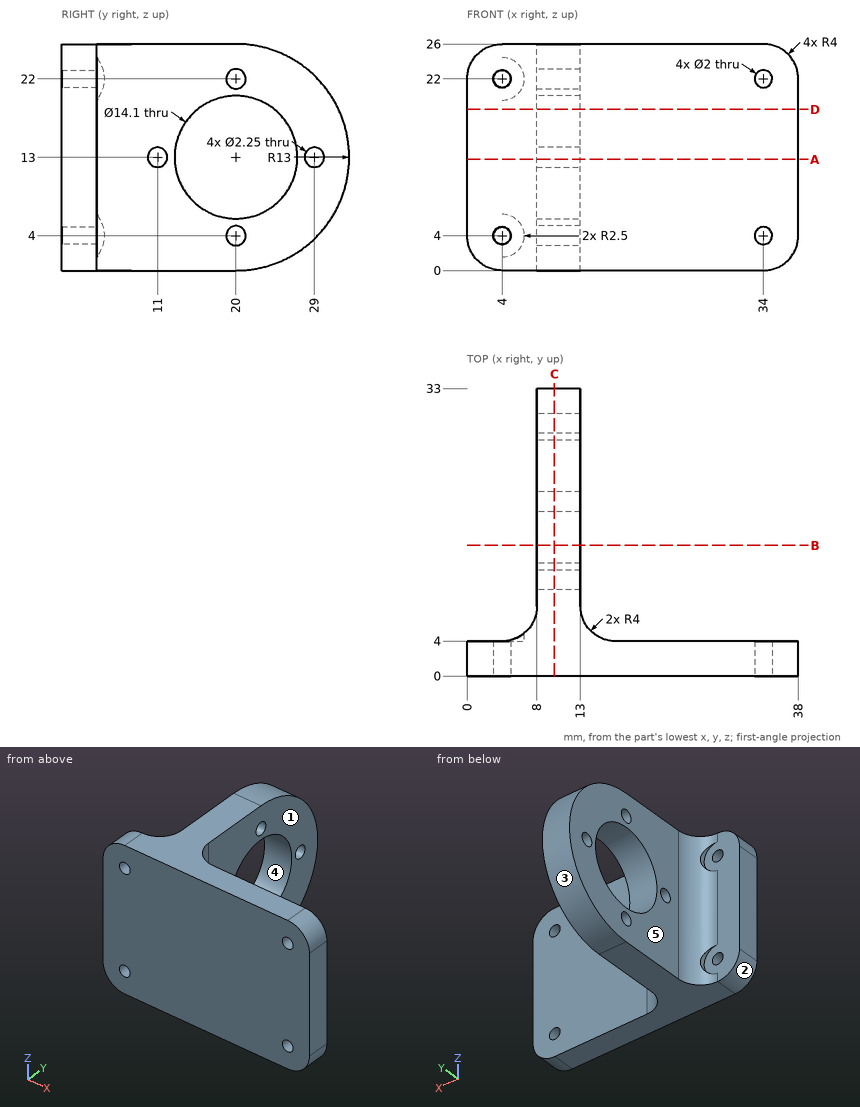
Here's the drawing with two shaded views (mm, measured from the low corner). I have some questions. A direction names the side the tool comes from. Round coordinates to 2 decimals unless told otherwise and drop trailing zeros. Order: outer loops, then holes, each group sorted by start corner. A loop starts at its lowest first (then second) coordinate and runs counter-clockwise, first axis right, second up. Notation, with made-up numbers: (85.5, 57) -> (98.5, 57) arc R17 cw to (98.5, 88) -> close; hole circle Ø1 at (16.25, 41.5). An arc over 180 degrees is marked (long way). Write each question's results on one line, items separated by ' | '. Start each with the question number.
Item 1: If we section it at C-C, the plane x = 10: Write out the boundary of the cut face in (y, z) (3 decimals), then the cut area to 3 significant figures.
Item 2: Thinking about a two-plate mould opening in Z: for the marked faces 3, 4 and 5, which applies, +Z half, -Z half, draft (parallel to the pull), parting line (faces both ways), or undercut?
Item 3: Which directions (+Z, -Z, +X, -X, +Y, -Y) give clear straight access to the entire face, cutting with the end or side of a thin tool? Please do the marked faces 1 and 2.
Item 4: Will these pins go through, and if not, where does the flat tip stop? pin 1 (10.5 mm diameter, centred on x = 23.5, z = 8.5, fed in from +Y); pin 2 (1.8 mm diameter, centred on x = 34, z = 4, fed in from -Y); pin 3 (3 mm diameter, centred on x = 10.5, z = 7.5, fed in from +Y); pin 4 (3 mm diameter, centred on y = 29.5, z = 17, fed in from -X).
Item 5: If we section it at D-D, the plane z = 18.5: Write out the boundary of the cut face in (x, y), then the cut area to 3 significant figures.
Item 6: If we section it at B-B, the plane y = 15: Write out the boundary of the cut face in (x, z), then the cut area to 3 significant figures.
Item 7: If we section it at A-A, the plane z = 12.75: Write out the boundary of the cut face in (x, y), then the cut area to 3 significant figures.
Item 8: Please list where these lines run through material, in increasing order: L1, parallel to Y at x = 10.5, z = 13 (3 decimals); L2, parallel to Y at x = 10, z = 12.5; L3, parallel to X at y = 26, z = 18.5.
Results:
1) outline: (0, 0) -> (20, 0) arc R13 ccw to (20, 26) -> (0, 26) -> close; hole circle Ø2.25 at (11, 13); hole circle Ø14.1 at (20, 13); hole circle Ø2.25 at (20, 4); hole circle Ø2.25 at (20, 22); hole circle Ø2.25 at (29, 13) | area: 613 mm2
2) face 3: parting line | face 4: undercut | face 5: draft
3) face 1: +Z, -Z, +X, +Y | face 2: -Z, -X, +Y, -Y
4) pin 1: stops at y = 4 | pin 2: passes through | pin 3: stops at y = 32.37 | pin 4: stops at x = 8
5) outline: (0, 0) -> (38, 0) -> (38, 4) -> (17, 4) arc R4 cw to (13, 8) -> (13, 15.59) -> (8, 15.59) -> (8, 8) arc R4 cw to (4, 4) -> (0, 4) -> close; (8, 24.41) -> (13, 24.41) -> (13, 31.78) -> (8, 31.78) -> close | area: 254 mm2
6) outline: (8, 0) -> (13, 0) -> (13, 8.03) -> (8, 8.03) -> close; (8, 17.97) -> (13, 17.97) -> (13, 26) -> (8, 26) -> close | area: 80.3 mm2
7) outline: (0, 0) -> (38, 0) -> (38, 4) -> (17, 4) arc R4 cw to (13, 8) -> (13, 9.9) -> (8, 9.9) -> (8, 8) arc R4 cw to (4, 4) -> (0, 4) -> close; (8, 12.1) -> (13, 12.1) -> (13, 12.95) -> (8, 12.95) -> close; (8, 27.05) -> (13, 27.05) -> (13, 27.9) -> (8, 27.9) -> close; (8, 30.1) -> (13, 30.1) -> (13, 33) -> (8, 33) -> close | area: 211 mm2
8) L1: y = 0 to 9.875, 12.125 to 12.95, 27.05 to 27.875, 30.125 to 33 | L2: y = 0 to 9.99, 12.01 to 12.97, 27.03 to 27.99, 30.01 to 32.99 | L3: x = 8 to 13
